Check sheet for the modelled part. Datum: model origin and axes. Units: mm. Face numbers are marked on the shaded views. A direction names the side the tool comes from. Coordinates: 2 decimals unless noted, no trailing zeros. Order: outer loops, then holes, each group sorted by start corner. A loop starts at its lowest first (then second) coordinate and runs counter-clockwise, first axis right, second up.
1. Set-up check for the marked faces 1 and 2: record each of +Z, -Z, +X, -X, +Y, -Y from which the full face is reachable in a straight line by a thin tool's end or side.
2. Thickness scan on line 1 (X direction, y = -12, z = -7); line 2 (Z direction, x = 1.25, y = 22); line 3 (Y direction, x = 2.25, z = -22.5). Record the ranges inside material, lowest first.
3. Cross-section at D-D (x = 3). Enter the section's corners in (y, z), then the cut area to 3 significant figures.
4. Cross-section at A-A (z = 0). Enter the section's corners in (x, y), then the cut area to 3 significant figures.
5. Cross-section at C-C (x = 13). Enter the section's corners in (y, z), then the cut area to 3 significant figures.
6. Gauge pin test, flat ends, axial feed: pin 1 Ø1 at (x, z) = (8, -19.5) entering from +Y; pin 2 Ø1.5 at (y, z) = (18, 18.5) entering from -X; pin 3 Ø5 at (y, z) = (14, -8) entering from +X; pin 4 Ø4 at (x, z) = (4, 9.5) entering from -Y. Record the tip position at first contact, or that the pin passes through.
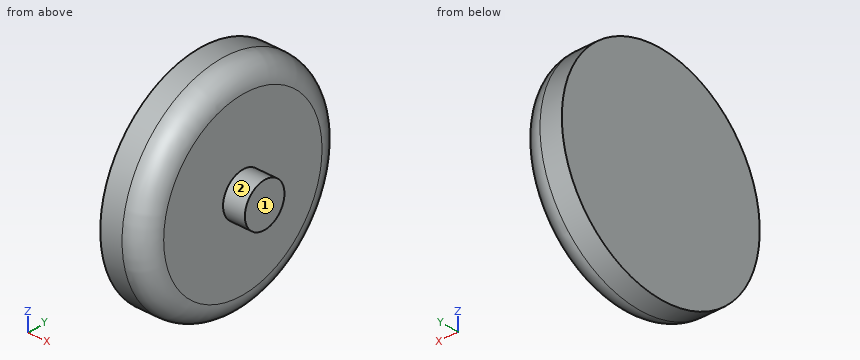
```python
from build123d import *

# Parameters (mm, degrees)
SKETCH1_R           = 25
BOSS_EXTRUDE1_DEPTH = 10
FILLET1_R           = 5
SKETCH2_R           = 5
BOSS_EXTRUDE2_DEPTH = 5


with BuildPart() as part:
    # Sketch1 → Boss-Extrude1 (new body)
    with BuildSketch(Plane(origin=(0, 0, 0), x_dir=(0, 0, -1), z_dir=(1, 0, 0))):
        Circle(SKETCH1_R)
    extrude(amount=BOSS_EXTRUDE1_DEPTH)

    # Fillet1
    fillet1_edges = [part.edges().sort_by_distance(p)[0] for p in [
        (10, 0, 25),
    ]]
    fillet(fillet1_edges, radius=FILLET1_R)

    # Sketch2 → Boss-Extrude2 (add)
    with BuildSketch(Plane(origin=(10, 0, 0), x_dir=(0, 0, -1), z_dir=(1, 0, 0))):
        Circle(SKETCH2_R)
    extrude(amount=BOSS_EXTRUDE2_DEPTH)


solid = part.part
```
Data:
1. face 1: +Z, -Z, +X, +Y, -Y
1. face 2: +X
2. line 1: x = 0 to 10
2. line 2: z = -11.87 to 11.87
2. line 3: y = -10.9 to 10.9
3. outline: circle Ø50 at (0, 0)
3. area: 1,960 mm2
4. outline: (0, -25) - (5, -25) arc R5 ccw to (10, -20) - (10, -5) - (15, -5) - (15, 5) - (10, 5) - (10, 20) arc R5 ccw to (5, 25) - (0, 25) - close
4. area: 539 mm2
5. outline: circle Ø10 at (0, 0)
5. area: 78.5 mm2
6. pin 1: stops at y = 14.87
6. pin 2: passes through
6. pin 3: stops at x = 10
6. pin 4: stops at y = -23.85
